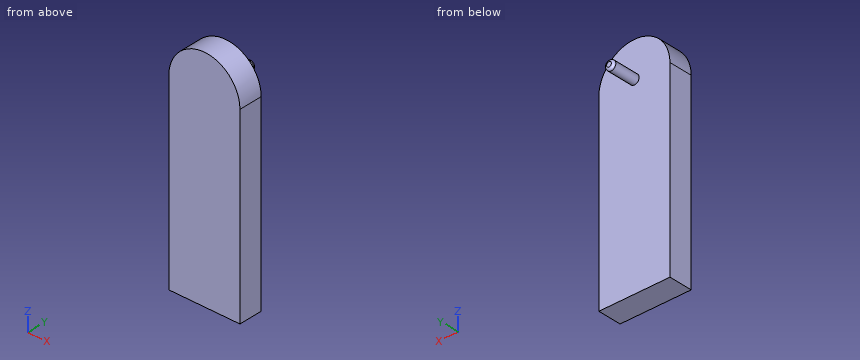
```python
from build123d import *

# Parameters (mm, degrees)
EXTRUDE_1_DEPTH = 50
SKETCH_2_R      = 10
EXTRUDE_2_DEPTH = 60
FILLET_1_R      = 5


with BuildPart() as part:
    # 草图1 → 凸台-拉伸1 (new body)
    with BuildSketch(Plane(origin=(0, 0, 0), x_dir=(1, 0, 0), z_dir=(0, 1, 0))):
        with BuildLine():
            Line((0, 0), (150, 0))
            Line((150, 0), (150, -400))
            ThreePointArc((150, -400), (75, -475), (0, -400))
            Line((0, -400), (0, 0))
        make_face()
    extrude(amount=EXTRUDE_1_DEPTH)

    # 草图2 → 凸台-拉伸2 (add)
    with BuildSketch(Plane(origin=(0, 50, 0), x_dir=(1, 0, 0), z_dir=(0, 1, 0))):
        with Locations((75, -400)):
            Circle(SKETCH_2_R)
    extrude(amount=EXTRUDE_2_DEPTH)

    # 圆角1
    fillet_1_edges = [part.edges().sort_by_distance(p)[0] for p in [
        (65, 110, 400),
    ]]
    fillet(fillet_1_edges, radius=FILLET_1_R)


solid = part.part
```
Geometry: final body of the model. Coordinates: model frame, mm. Round coordinates to 2 decimals unless told otherwise and drop trailing zeros. Order: outer loops, then holes, each group sorted by start corner. A loop starts at its lowest first (then second) coordinate and runs counter-clockwise, first axis right, second up. Notation, with made-up numbers: (-35, -13.75) - (18, -13.75) arc R4 cw to (18, -7.75) - close; hole circle Ø1 at (-33.75, 0.25). An arc over 180 degrees is marked (long way). Write item = value, one per line. Start each with the question number.
Q1. Cut plane A-A on z = 85. Return the cut outline in (x, y).
Q2. Cut plane B-B on y = 10.5. Return the cut outline in (x, z), and give its area (3 significant figures).
Q3. Pin query (flat end, axial travel): pin 1 (8 mm diameter, centred on x = 61, z = 363, fed in from +Y); pin 2 (10 mm diameter, centred on x = 18, y = 33, fed in from +Z). Return the tip coordinate at first contact, or that it passes through.
Q4. Ray query, line 1 (Y direction, x = 124.5, z = 140.5); line 2 (Z direction, x = 76, y = 103); line 3 (Z direction, x = 22, y = 44). Return the intervals inside material, ascending. Write a range as from..to.
Outcome:
q1.outline = (0, 0) - (150, 0) - (150, 50) - (0, 50) - close
q2.outline = (0, 0) - (150, 0) - (150, 400) arc R75 ccw to (0, 400) - close
q2.area = 68,800 mm^2
q3.pin_1 = 50
q3.pin_2 = 454.05
q4.line_1 = 0..50
q4.line_2 = 390.05..409.95
q4.line_3 = 0..453.07
